Here's the drawing with two shaded views (mm, measured from the low corner). I have some questions. A direction names the side the tool comes from. Give positions to 0.01 mm unless a question says otherwise; leave off trailing zeros. Loops run counter-clockwise (first coordinate to the right, second up) from the corner with the lowest first, then second, coordinate; pieces in that order, holes last. Notation, with made-up numbers: (46.5, 32) - (67.5, 32) arc R19 cw to (67.5, 51) - close; hole circle Ø6 at (66, 86.5). An arc over 180 degrees is marked (long way). Use a Markdown table: item, result. Add a question column.
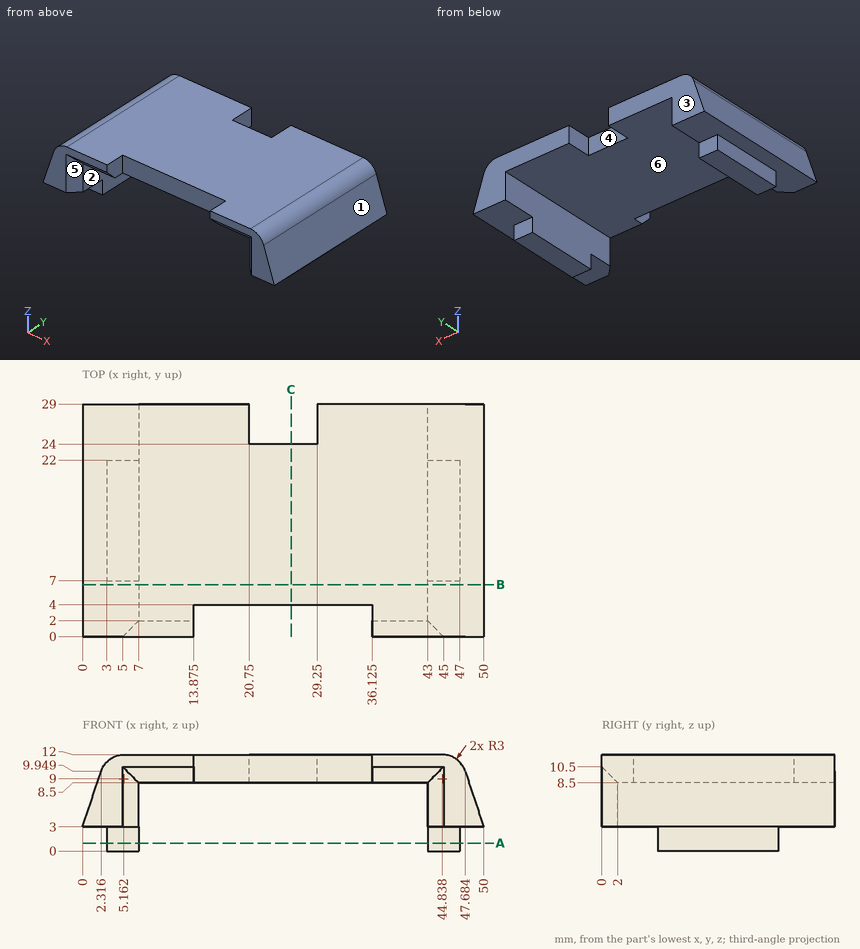
1. Suppose I cut it at C-C (x = 26). List the corners of the cut face in (y, z) for me, and give its area (3 significant figures).
2. Suppose I cut it at B-B (y = 6.5). List the corners of the cut face in (x, z) for me.
3. On a 3-axis mill with a long thin cutter (end or side, diameter ignored), from which of +Z, -Z, +X, -X, +Y, -Y can I reach the whole of each face in a straight line? I mean the marked faces 4, 5 and 6. Say none if no direction works.
4. Will these pins go through, and if not, where does the flat tip stop? P1, Ø3, axis at x = 25, z = 9.5, coming from the -Y side; P2, Ø1.5, axis at x = 46, z = 1.5, coming from the -Y side; P3, Ø8, axis at x = 22.5, y = 21.5, coming from the -Z side.
5. Please list where these lines run through material, in increasing order: line 1 along X through (y, z) = (7.25, 1.75); line 2 along Z through (x, y) = (32, 11); line 3 along Z through (x, y) = (6.5, 25.5). Write a range as [from, to].
6. If we mould it in two halves opening along X, with no side actions, what happens to the marked faces 1, 2 and 3? For each: released by +X, released by -X, zero draft, split by the parting line, or undercut.
7. Suppose I cut it at A-A (z = 1). List the corners of the cut face in (x, y) for me, and give its area (3 significant figures).
Results below:
| question | item | result |
|---|---|---|
| 1 | outline | (4, 8.5) - (24, 8.5) - (24, 12) - (4, 12) - close |
| 1 | area | 70.0 mm² |
| 2 | outline | (0, 3) - (7, 3) - (7, 8.5) - (43, 8.5) - (43, 3) - (50, 3) - (47.68, 9.95) arc R3 ccw to (44.84, 12) - (5.16, 12) arc R3 ccw to (2.32, 9.95) - close |
| 3 | face 4 | +Z, -Z, +Y |
| 3 | face 5 | -Z, -Y |
| 3 | face 6 | -Z, +Y, -Y |
| 4 | P1 | y = 4 |
| 4 | P2 | y = 7 |
| 4 | P3 | z = 8.5 |
| 5 | line 1 | [3, 7], [43, 47] |
| 5 | line 2 | [8.5, 12] |
| 5 | line 3 | [3, 12] |
| 6 | face 1 | released by +X |
| 6 | face 2 | undercut |
| 6 | face 3 | zero draft |
| 7 | outline | (3, 7) - (7, 7) - (7, 22) - (3, 22) - close; (43, 7) - (47, 7) - (47, 22) - (43, 22) - close |
| 7 | area | 120 mm² |
